Check sheet for the drawn part. Datum: minimum x, y, z corner. Units: mm. A direction names the side the tool comes from. Give positions to 0.01 mm unless a question says otherwise; leave off trailing zeros. Write each loop counter-clockwise with the first axis right and the second up, starting at its lowest first coordinate (ties: lowest second). Pieces come first, ordered by that corner, then holes. Notation, with made-up numbers: M 87.25,71 L 144.25,71 A24 cw 144.25,103 Z; hole C 77,20.25 d10. An arc over 180 degrees is marked long. Use CSV: the item, a comma, the result in double quotes. Start each with the question number.
1. Cross-section at B-B, the plane z = 15.75. Enter the section's corners in (x, y) (1 decimal).
2. Scan lines: line 1 (X direction, y = 10.75, z = 16.5) (1 decimal); line 2 (Z direction, x = 1.75, y = 22.5). Record each from-to range of solid material in increasing order.
3. Cross-section at D-D, the plane x = 9.75. Enter the section's corners in (y, z) (1 decimal).
4. Depth check by flat-ended pin: P1, Ø1.4, axis at x = 6.85, y = 19.05, coming from the +Z side; P2, Ø1, axis at y = 10, z = 6.5, coming from the +X side (3 decimals); P3, Ø3.5, axis at x = 16, z = 2, coming from the +Y side; P4, Ø1.6, axis at y = 20.5, z = 1, coming from the +X side. Enter the tip coordinate at first touch or a pass-through.
5. Access from +Z, -Z, +X, -X, +Y, -Y to the whole of each face (thin tool, end or side, straight path). Record for the marked faces 1, 2 and 3.
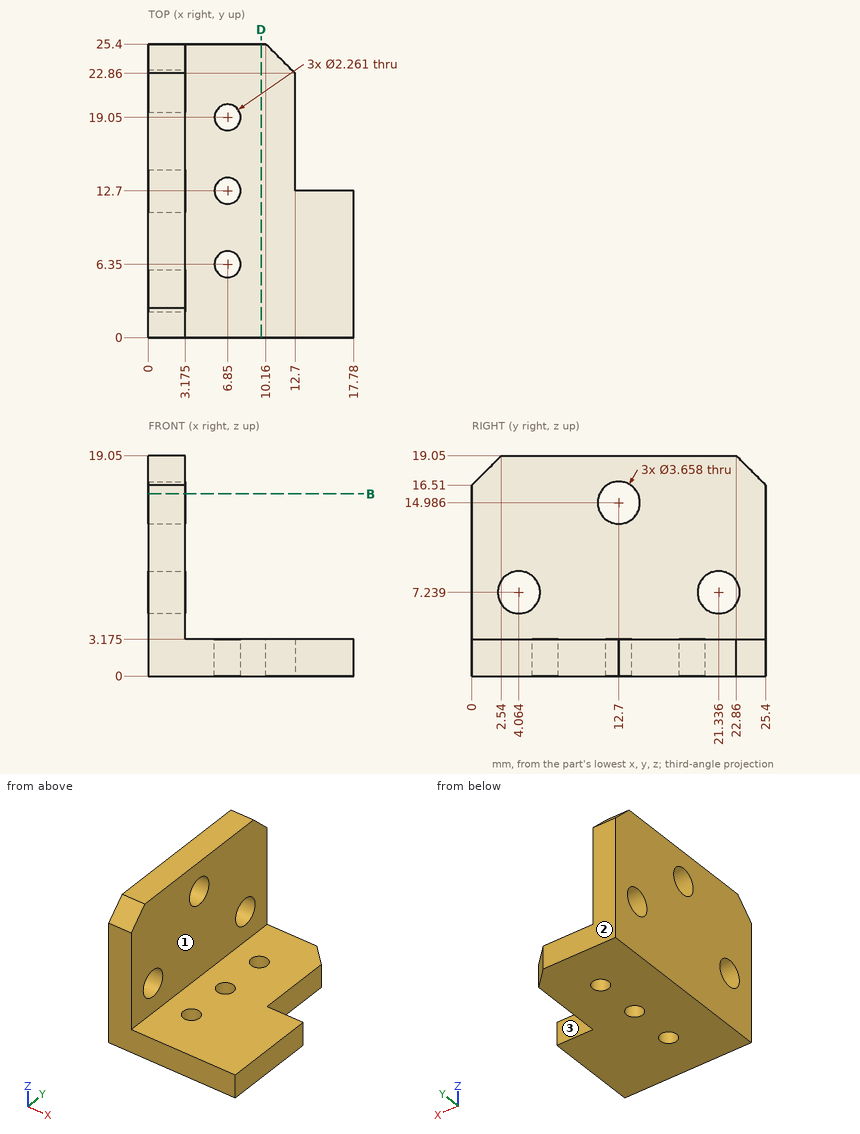
Worked answers:
1,outline,"M 0,0 L 3.2,0 L 3.2,11 L 0,11 Z; M 0,14.4 L 3.2,14.4 L 3.2,25.4 L 0,25.4 Z"
2,line 1,"x = 0 to 3.2"
2,line 2,"z = 0 to 5.83, 8.65 to 19.05"
3,outline,"M 0,0 L 25.4,0 L 25.4,3.2 L 0,3.2 Z"
4,P1,"passes through"
4,P2,"stops at x = 3.175"
4,P3,"stops at y = 12.7"
4,P4,"stops at x = 12.7"
5,face 1,"+Z, +X, +Y, -Y"
5,face 2,"+Z, -Z, +X, -X, +Y"
5,face 3,"+Z, -Z, +X, +Y"
